Model file for the job. Use its own axes, mm. A direction names the side the tool comes from. Round coordinates to 2 decimals unless told otherwise and drop trailing zeros. Loops run counter-clockwise (first coordinate to the right, second up) from the corner with the lowest first, then second, coordinate; pieces in that order, holes last. Notation, with made-up numbers: M -16.5,37.25 L 14.5,37.25 A8 cw 14.5,43.25 Z; hole C -4,-14.5 d4. An arc over 180 degrees is marked long. Use a Markdown table: item, result. Add a question column.
Item 1: Saw through at C-C on x = -49.5. Write the cut outline in (y, z), then the cut area to 3 significant figures.
Item 2: Wall check: L1, parallel to Z at x = 0.35, y = 6.35 (3 decimals); L2, parallel to X at y = 3.25, z = -61.5; L3, parallel to Y at x = -67.85, z = -146.05 (3 decimals). Give the ranges that are in metal, low to high. Write a range as from..to.
Item 3: Tool access for faces 1 (the flat face through (-28, 1, -152.4)), 2 (the flat face through (-34, 1.27, -75)): list every direction of +Z, -Z, +X, -X, +Y, -Y with a clear straight run to the whole face (end or side of a thin tool).
Item 4: Saw through at A-A on z = -48. Write the cut outline in (x, y) (3 decimals), then the cut area to 3 significant figures.
Item 5: Saw through at B-B on y = 5. Write the cut outline in (x, z).
Item 6: Pin check, flat tips, straight feed: P1, Ø5.5, axis at y = 6.35, z = -6.35, coming from the +X side; P2, Ø3, axis at x = -44.5, y = 1.5, coming from the -Z side; P3, Ø12, axis at x = -16, z = -107, coming from the +Y side. Stop position of each tip, or through.
Item 7: Two-plate mould, pull along Y, no slides. Class faces 3 (the cylindrical face through (-67.94, 10.89, -1.91)), 4 (the flat face through (0, 7, -75)), 5 (the cylindrical face through (-67.94, 5.94, -142.9)): +Y half, -Y half, draft (parallel to the pull), parting line (faces both ways), or undercut.
```python
from build123d import *

# Parameters (mm, degrees)
F0_R     = 3.175
F1_DEPTH = 1.27
F3_DEPTH = 152.4


with BuildPart() as f1:
    # F0 (on Right) → F1 (new body)
    with BuildSketch(Plane.YZ):
        with BuildLine():
            Line((6.35, 0), (0, 0))
            Line((0, 0), (0, -76.2))
            Line((0, -76.2), (12.7, -76.2))
            Line((12.7, -76.2), (12.7, -6.35))
            ThreePointArc((12.7, -6.35), (10.840128, -1.859872), (6.35, 0))
        make_face()
        with Locations((6.35, -6.35)):
            Circle(F0_R, mode=Mode.SUBTRACT)
        with BuildLine():
            Line((12.7, -76.2), (0, -76.2))
            Line((0, -76.2), (0, -152.4))
            Line((0, -152.4), (6.35, -152.4))
            ThreePointArc((6.35, -152.4), (10.840128, -150.540128), (12.7, -146.05))
            Line((12.7, -146.05), (12.7, -76.2))
        make_face()
        with Locations((6.35, -146.05)):
            Circle(F0_R, mode=Mode.SUBTRACT)
    extrude(amount=F1_DEPTH)

    # F2 (on face) → F3 (join, through all)
    with BuildSketch(Plane.XY):
        with BuildLine():
            ThreePointArc((0, 1.905), (-0.185987, 1.455987), (-0.635, 1.27))
            Line((-0.635, 1.27), (-33.655, 1.27))
            Line((-33.655, 1.27), (-33.655, 0))
            Line((-33.655, 0), (0, 0))
            Line((0, 0), (0, 1.905))
        make_face()
    extrude(amount=-F3_DEPTH)

    # F4: F1 across face


with BuildPart() as f1_1:
    add(f1.part)
    add(f1.part.mirror(Plane(origin=(-33.655, 0.635, -76.2), x_dir=(0, -1, 0), z_dir=(-1, 0, 0))))


solid = f1_1.part
```
Entries:
| question | item | result |
|---|---|---|
| 1 | outline | M 0,-152.4 L 1.27,-152.4 L 1.27,0 L 0,0 Z |
| 1 | area | 194 mm2 |
| 2 | L1 | -152.4..-149.225, -142.875..-9.525, -3.175..0 |
| 2 | L2 | -68.58..-67.31, 0..1.27 |
| 2 | L3 | 0..3.175, 9.525..12.7 |
| 3 | face 1 | -Z, +X, -X, +Y, -Y |
| 3 | face 2 | +Z, -Z, +Y |
| 4 | outline | M -68.58,0 L 1.27,0 L 1.27,12.7 L 0,12.7 L 0,1.905 A0.635 cw -0.635,1.27 L -66.675,1.27 A0.635 cw -67.31,1.905 L -67.31,12.7 L -68.58,12.7 Z |
| 4 | area | 118 mm2 |
| 5 | outline | M -68.58,-152.4 L -67.31,-152.4 L -67.31,-148.92 L -68.58,-148.92 Z; M -68.58,-143.18 L -67.31,-143.18 L -67.31,-9.22 L -68.58,-9.22 Z; M -68.58,-3.48 L -67.31,-3.48 L -67.31,0 L -68.58,0 Z; M 0,-152.4 L 1.27,-152.4 L 1.27,-148.92 L 0,-148.92 Z; M 0,-143.18 L 1.27,-143.18 L 1.27,-9.22 L 0,-9.22 Z; M 0,-3.48 L 1.27,-3.48 L 1.27,0 L 0,0 Z |
| 6 | P1 | through |
| 6 | P2 | z = -152.4 |
| 6 | P3 | y = 1.27 |
| 7 | face 3 | +Y half |
| 7 | face 4 | draft |
| 7 | face 5 | undercut |
